Read the model definition and answer for the solid it produces. Units are mm, in the model's axes. A direction names the side the tool comes from. Give positions to 0.01 mm unless a question says otherwise; leave off trailing zeros. Write each loop counter-clockwise with the first axis right and the second up, starting at its lowest first coordinate (ties: lowest second). Pieces come first, ordered by that corner, then holes. Notation, with made-up numbers: M -39,-22.75 L -20,-22.75 A20 cw -20,-8.75 Z; hole C 36,-2.5 d6. An arc over 180 degrees is marked long. Use a Markdown table: item, result. Add a question column.
Item 1: A cutting plane is placed at A-A on y = 4.75. Determine the outline of the cut face in (x, z), then the cut area to 3 significant figures.
Item 2: Consider probe 1 along Y at (x, z) = (0, 1.3); probe 2 along Z at (x, y) = (0, -23.9); probe 3 along Y at (x, z) = (23, 35). Determine where each line is inside the solid, lowest interval first. Write a range as [from, to].
Item 3: For faces 1 (the flat face through (0, -24, 53.5)), 2 (the flat face through (11.356, -9.081, 1.232)), 3 (the flat face through (0, -9, 2.5)), determine the directions among +Z, -Z, +X, -X, +Y, -Y from which every point of the face is accessible in a straight line to the end or side of a thin tool.
Item 4: Given P1, Ø5, axis at x = 3, y = -20, coming from the +Z side; P2, Ø5, axis at x = 0, z = 40, coming from the +Y side; P3, Ø12, axis at x = 3.5, y = 14.5, coming from the -Z side, each flat-ended and moving along its own axis, determine where each tip first touches the part or whether it passes through.
Item 5: A cutting plane is placed at D-D on x = 18.5. Determine the outline of the cut face in (y, z).
Item 6: The mould has two halves that part along X. Classify faces 4 (the cylindrical face through (-16.087, 3.533, 1.232)), 5 (the cylindrical face through (8.28, 13.09, 1.23)), 6 (the flat face through (0, -23.25, 28)), 7 (the flat face through (22.5, -24.5, 51)): pulls with the +X half, pulls with the -X half, needs draft (parallel to the pull), parting line crosses it, or undercut.
Item 7: A cutting plane is placed at C-C on x = 0. Determine the outline of the cut face in (y, z), then the cut area to 3 significant figures.
Item 8: A cutting plane is placed at B-B on z = 40. Determine the outline of the cut face in (x, y), then the cut area to 3 significant figures.
from build123d import *

# Parameters (mm, degrees)
SKETCH_14_W         = 50
SKETCH_14_H         = 51.5
SKETCH_14_R         = 11
SKETCH_14_R_2       = 2
EXTRUDE_1_DEPTH     = 2.5
SKETCH_16_W         = 50
SKETCH_16_H         = 2.5
EXTRUDE_2_DEPTH     = 51
SKETCH_17_R         = 2.15
CUT_EXTRUDE_1_DEPTH = 3.5
CHAMFER_1_SIZE      = 5


with BuildPart() as part:
    # 草图14 → 凸台-拉伸1 (new body)
    with BuildSketch(Plane.XY):
        Rectangle(SKETCH_14_W, SKETCH_14_H)
        with Locations((0, 4.75)):
            Circle(SKETCH_14_R, mode=Mode.SUBTRACT)
        with Locations((-14.5, 4.75)):
            Circle(SKETCH_14_R_2, mode=Mode.SUBTRACT)
        with Locations((14.5, 4.75)):
            Circle(SKETCH_14_R_2, mode=Mode.SUBTRACT)
        with BuildLine():
            Line((-14.318912319, 21.543786053), (-8.308504679, 15.533378413))
            ThreePointArc((-8.308504679, 15.533378413), (-8.308504679, 13.058504679), (-10.783378413, 13.058504679))
            Line((-10.783378413, 13.058504679), (-16.793786053, 19.068912319))
            ThreePointArc((-16.793786053, 19.068912319), (-16.793786053, 21.543786053), (-14.318912319, 21.543786053))
        make_face(mode=Mode.SUBTRACT)
        with BuildLine():
            Line((14.318912319, 21.543786053), (8.308504679, 15.533378413))
            ThreePointArc((8.308504679, 15.533378413), (8.308504679, 13.058504679), (10.783378413, 13.058504679))
            Line((10.783378413, 13.058504679), (16.793786053, 19.068912319))
            ThreePointArc((16.793786053, 19.068912319), (16.793786053, 21.543786053), (14.318912319, 21.543786053))
        make_face(mode=Mode.SUBTRACT)
        with BuildLine():
            Line((-14.318912319, -12.043786053), (-8.308504679, -6.033378413))
            ThreePointArc((-8.308504679, -6.033378413), (-8.308504679, -3.558504679), (-10.783378413, -3.558504679))
            Line((-10.783378413, -3.558504679), (-16.793786053, -9.568912319))
            ThreePointArc((-16.793786053, -9.568912319), (-16.793786053, -12.043786053), (-14.318912319, -12.043786053))
        make_face(mode=Mode.SUBTRACT)
        with BuildLine():
            Line((14.318912319, -12.043786053), (8.308504679, -6.033378413))
            ThreePointArc((8.308504679, -6.033378413), (8.308504679, -3.558504679), (10.783378413, -3.558504679))
            Line((10.783378413, -3.558504679), (16.793786053, -9.568912319))
            ThreePointArc((16.793786053, -9.568912319), (16.793786053, -12.043786053), (14.318912319, -12.043786053))
        make_face(mode=Mode.SUBTRACT)
    extrude(amount=EXTRUDE_1_DEPTH)

    # 草图16 → 凸台-拉伸2 (add)
    with BuildSketch(Plane.XY.offset(2.5)):
        with Locations((0, -24.5)):
            Rectangle(SKETCH_16_W, SKETCH_16_H)
    extrude(amount=EXTRUDE_2_DEPTH)

    # 草图17 → 切除-拉伸1 (cut, through all)
    with BuildSketch(Plane(origin=(0, -23.25, 0), x_dir=(1, 0, 0), z_dir=(0, 1, 0))):
        with Locations((0, -40)):
            Circle(SKETCH_17_R)
        with Locations((0, -16)):
            Circle(SKETCH_17_R)
    extrude(amount=-CUT_EXTRUDE_1_DEPTH, mode=Mode.SUBTRACT)

    # 倒角1
    chamfer_1_edges = [part.edges().sort_by_distance(p)[0] for p in [
        (-25, 25.75, 1.25),
        (25, 25.75, 1.25),
        (-25, -24.5, 53.5),
        (25, -24.5, 53.5),
    ]]
    chamfer(chamfer_1_edges, length=CHAMFER_1_SIZE)


solid = part.part
Filled in:
| question | item | result |
|---|---|---|
| 1 | outline | M -25,0 L -16.5,0 L -16.5,2.5 L -25,2.5 Z; M -12.5,0 L -11,0 L -11,2.5 L -12.5,2.5 Z; M 11,0 L 12.5,0 L 12.5,2.5 L 11,2.5 Z; M 16.5,0 L 25,0 L 25,2.5 L 16.5,2.5 Z |
| 1 | area | 50.0 mm² |
| 2 | probe 1 | [-25.75, -6.25], [15.75, 25.75] |
| 2 | probe 2 | [0, 13.85], [18.15, 37.85], [42.15, 53.5] |
| 2 | probe 3 | [-25.75, -23.25] |
| 3 | face 1 | +Z, +X, -X, +Y, -Y |
| 3 | face 2 | +Z, -Z |
| 3 | face 3 | +Z, +X, -X, +Y |
| 4 | P1 | z = 2.5 |
| 4 | P2 | y = -23.25 |
| 4 | P3 | z = 0 |
| 5 | outline | M -25.75,0 L 25.75,0 L 25.75,2.5 L -23.25,2.5 L -23.25,53.5 L -25.75,53.5 Z |
| 6 | face 4 | undercut |
| 6 | face 5 | undercut |
| 6 | face 6 | needs draft |
| 6 | face 7 | pulls with the +X half |
| 7 | outline | M -25.75,0 L -6.25,0 L -6.25,2.5 L -23.25,2.5 L -23.25,13.85 L -25.75,13.85 Z; M -25.75,18.15 L -23.25,18.15 L -23.25,37.85 L -25.75,37.85 Z; M -25.75,42.15 L -23.25,42.15 L -23.25,53.5 L -25.75,53.5 Z; M 15.75,0 L 25.75,0 L 25.75,2.5 L 15.75,2.5 Z |
| 7 | area | 180 mm² |
| 8 | outline | M -25,-25.75 L -2.15,-25.75 L -2.15,-23.25 L -25,-23.25 Z; M 2.15,-25.75 L 25,-25.75 L 25,-23.25 L 2.15,-23.25 Z |
| 8 | area | 114 mm² |
